CAD build for the part. Positions are in the model's coordinates, mm. Face numbers are marked on the shaded views. Give positions to 0.01 mm unless a question says otherwise; leave off trailing zeros. Write each loop counter-clockwise with the first axis right and the second up, starting at its lowest first coordinate (ties: lowest second). Pieces come first, ordered by that corner, then holes. Notation, with made-up numbers: (29, -9.5) -> (65, -9.5) arc R23 ccw to (65, 6.5) -> close; hole circle Ø8 at (7, 58.25). An arc over 180 degrees is marked (long way). Answer as a JSON object with one key per item and string values.
```python
from build123d import *

# Parameters (mm, degrees)
ESQUISSE1_R             = 3.5
BASE_EXTRUSION_DEPTH    = 4
ESQUISSE2_R             = 2
BOSS_EXTRU_1_DEPTH      = 16
ENL_V_MAT_EXTRU_1_DEPTH = 4
CONG_1_R                = 0.5
CHANFREIN1_SIZE         = 0.5


with BuildPart() as part:
    # Esquisse1 → Base-Extrusion (new body)
    with BuildSketch(Plane.XY):
        Circle(ESQUISSE1_R)
    extrude(amount=BASE_EXTRUSION_DEPTH)

    # Esquisse2 → Boss.-Extru.1 (add)
    with BuildSketch(Plane(origin=(0, 0, 0), x_dir=(-1, 0, 0), z_dir=(0, 0, -1))):
        Circle(ESQUISSE2_R)
    extrude(amount=BOSS_EXTRU_1_DEPTH)

    # Esquisse3 → Enlèv. mat.-Extru.1 (cut)
    with BuildSketch(Plane.XY.offset(4)):
        Polygon((1.884038216, 0), (0.744038216, 1.5), (-0.744038216, 1.5), (-1.884038216, 0), (-0.744038216, -1.5), (0.744038216, -1.5), align=None)
    extrude(amount=-ENL_V_MAT_EXTRU_1_DEPTH, mode=Mode.SUBTRACT)

    # Congé1
    cong_1_edges = [part.edges().sort_by_distance(p)[0] for p in [
        (-3.5, 0, 4),
    ]]
    fillet(cong_1_edges, radius=CONG_1_R)

    # Chanfrein1
    chanfrein1_edges = [part.edges().sort_by_distance(p)[0] for p in [
        (2, 0, -16),
    ]]
    chamfer(chanfrein1_edges, length=CHANFREIN1_SIZE)


solid = part.part
```
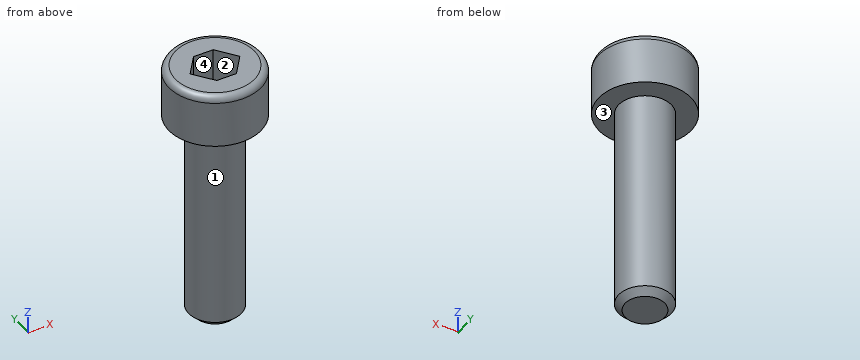
1) Slice it at C-C (z = -5.75). List the corners of the cut face in (x, y), then the cut area to 3 significant figures.
Model answer:
{"outline": "circle Ø4 at (0, 0)", "area": "12.6 mm2"}
2) Mould opens along Y. For the marked faces 1, 2, 3 and 4 say: released by +Y, released by -Y, zero draft, split by the parting line, or undercut.
Model answer:
{"face 1": "split by the parting line", "face 2": "undercut", "face 3": "zero draft", "face 4": "undercut"}
3) Slice it at B-B (z = 1). List the corners of the cut face in (x, y), then the cut area to 3 significant figures.
Model answer:
{"outline": "circle Ø7 at (0, 0); hole (-1.88, 0) -> (-0.74, -1.5) -> (0.74, -1.5) -> (1.88, 0) -> (0.74, 1.5) -> (-0.74, 1.5) -> close", "area": "30.6 mm2"}
4) Wall check: probe 1 along Z at (x, y) = (-0.25, 0.25); probe 2 along Z at (x, y) = (-1.5, -2); probe 3 along X at (y, z) = (1.25, 1.5). Give the ranges that are in metal, low to high.
Model answer:
{"probe 1": "z = -16 to 0", "probe 2": "z = 0 to 4", "probe 3": "x = -3.27 to -0.93, 0.93 to 3.27"}
5) Pin check, flat tips, straight feed: pin 1 (0.9 mm diameter, centred on x = 0, y = 0, fed in from +Z); pin 2 (1 mm diameter, centred on x = 1.5, z = -13.5, fed in from -Y). Stop position of each tip, or through.
Model answer:
{"pin 1": "stops at z = 0", "pin 2": "stops at y = -1.73"}
6) Slice it at A-A (x = 0). List the corners of the cut face in (y, z).
Model answer:
{"outline": "(-3.5, 0) -> (-2, 0) -> (-2, -15.5) -> (-1.5, -16) -> (1.5, -16) -> (2, -15.5) -> (2, 0) -> (3.5, 0) -> (3.5, 3.5) arc R0.5 ccw to (3, 4) -> (1.5, 4) -> (1.5, 0) -> (-1.5, 0) -> (-1.5, 4) -> (-3, 4) arc R0.5 ccw to (-3.5, 3.5) -> close"}
